from build123d import *

# Parameters (mm, degrees)
SKETCH1_W           = 250
SKETCH1_H           = 127
BOSS_EXTRUDE1_DEPTH = 6.35
SKETCH2_R           = 6.35
SKETCH2_R_2         = 3.175
SKETCH2_R_3         = 9.525
SKETCH2_R_4         = 4
SKETCH2_R_5         = 12.5
CUT_EXTRUDE1_DEPTH  = 281.480520714
CUT_EXTRUDE2_DEPTH  = 281.480520714
SKETCH9_W           = 40.64
SKETCH9_H           = 25.4
CUT_EXTRUDE3_DEPTH  = 281.480520714
FILLET1_R           = 3.96875


with BuildPart() as part:
    # Sketch1 → Boss-Extrude1 (new body)
    with BuildSketch(Plane(origin=(0, 0, 0), x_dir=(1, 0, 0), z_dir=(0, 1, 0))):
        with Locations((125, 63.5)):
            Rectangle(SKETCH1_W, SKETCH1_H)
    extrude(amount=BOSS_EXTRUDE1_DEPTH)

    # Sketch2 → Cut-Extrude1 (cut, through all)
    with BuildSketch(Plane(origin=(0, 6.35, 0), x_dir=(1, 0, 0), z_dir=(0, 1, 0))):
        with Locations(Location((237.3, 12.7, 0), (0, 0, 270))):
            Circle(SKETCH2_R)
        with Locations(Location((237.3, 114.3, 0), (0, 0, 270))):
            Circle(SKETCH2_R)
        with Locations(Location((12.7, 12.7, 0), (0, 0, 270))):
            Circle(SKETCH2_R)
        with Locations(Location((12.7, 114.3, 0), (0, 0, 270))):
            Circle(SKETCH2_R)
        with Locations(Location((43.193581925, 36.693581925, 0), (0, 0, 270))):
            Circle(SKETCH2_R_2)
        with Locations(Location((96.806418075, 36.693581925, 0), (0, 0, 270))):
            Circle(SKETCH2_R_2)
        with Locations(Location((96.806418075, 90.306418075, 0), (0, 0, 270))):
            Circle(SKETCH2_R_2)
        with Locations(Location((43.193581925, 90.306418075, 0), (0, 0, 270))):
            Circle(SKETCH2_R_2)
        with Locations(Location((70, 63.5, 0), (0, 0, 270))):
            Circle(SKETCH2_R_3)
        with Locations(Location((105.55, 19.05, 0), (0, 0, 270))):
            Circle(SKETCH2_R_4)
        with Locations(Location((194.45, 19.05, 0), (0, 0, 270))):
            Circle(SKETCH2_R_4)
        with Locations(Location((194.45, 107.95, 0), (0, 0, 270))):
            Circle(SKETCH2_R_4)
        with Locations(Location((105.55, 107.95, 0), (0, 0, 270))):
            Circle(SKETCH2_R_4)
        with Locations(Location((150, 63.5, 0), (0, 0, 270))):
            Circle(SKETCH2_R_5)
    extrude(amount=-CUT_EXTRUDE1_DEPTH, mode=Mode.SUBTRACT)

    # Sketch8 → Cut-Extrude2 (cut, through all)
    with BuildSketch(Plane(origin=(0, 6.35, 0), x_dir=(1, 0, 0), z_dir=(0, 1, 0))):
        with BuildLine():
            Line((103.01, 111.95), (118.25, 111.95))
            ThreePointArc((118.25, 111.95), (122.25, 107.95), (118.25, 103.95))
            Line((118.25, 103.95), (103.01, 103.95))
            ThreePointArc((103.01, 103.95), (99.01, 107.95), (103.01, 111.95))
        make_face()
        with BuildLine():
            Line((191.91, 111.95), (207.15, 111.95))
            ThreePointArc((207.15, 111.95), (211.15, 107.95), (207.15, 103.95))
            Line((207.15, 103.95), (191.91, 103.95))
            ThreePointArc((191.91, 103.95), (187.91, 107.95), (191.91, 111.95))
        make_face()
        with BuildLine():
            Line((103.01, 23.05), (118.25, 23.05))
            ThreePointArc((118.25, 23.05), (122.25, 19.05), (118.25, 15.05))
            Line((118.25, 15.05), (103.01, 15.05))
            ThreePointArc((103.01, 15.05), (99.01, 19.05), (103.01, 23.05))
        make_face()
        with BuildLine():
            Line((191.91, 23.05), (207.15, 23.05))
            ThreePointArc((207.15, 23.05), (211.15, 19.05), (207.15, 15.05))
            Line((207.15, 15.05), (191.91, 15.05))
            ThreePointArc((191.91, 15.05), (187.91, 19.05), (191.91, 23.05))
        make_face()
    extrude(amount=-CUT_EXTRUDE2_DEPTH, mode=Mode.SUBTRACT)

    # Sketch9 → Cut-Extrude3 (cut, through all)
    with BuildSketch(Plane(origin=(0, 6.35, 0), x_dir=(1, 0, 0), z_dir=(0, 1, 0))):
        with Locations((155.08, 63.5)):
            Rectangle(SKETCH9_W, SKETCH9_H)
    extrude(amount=-CUT_EXTRUDE3_DEPTH, mode=Mode.SUBTRACT)

    # Fillet1
    fillet1_edges = [part.edges().sort_by_distance(p)[0] for p in [
        (134.76, 3.175, -50.8),
        (134.76, 3.175, -76.2),
        (175.4, 3.175, -76.2),
        (175.4, 3.175, -50.8),
    ]]
    fillet(fillet1_edges, radius=FILLET1_R)


solid = part.part
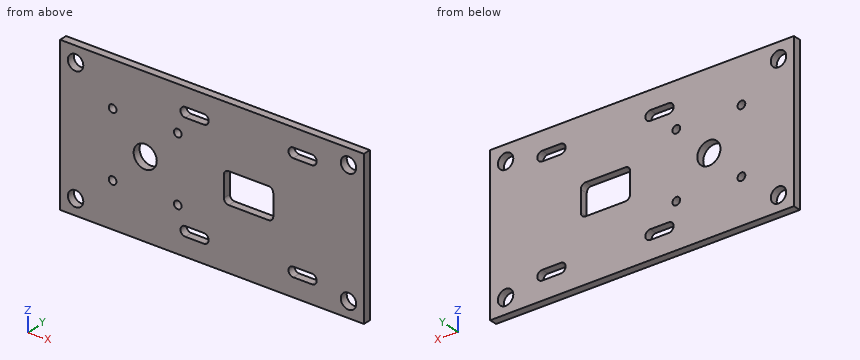
Work out the finished part from the listing and answer in its coordinate system (mm). Round coordinates to 2 decimals unless told otherwise and drop trailing zeros. Order: outer loops, then holes, each group sorted by start corner. A loop starts at its lowest first (then second) coordinate and runs counter-clockwise, first axis right, second up. Notation, with made-up numbers: M 88,-4 L 116,-4 A5 cw 116,5 Z; hole C -15,14 d1. An arc over 180 degrees is marked long. Put each result on its own line as item: value. Start each with the question number.
Q1. A flat-ended cylindrical pin translates along its axis: pin 1 (11.5 mm diameter, centred on x = 237.3, z = -114.3, fed in from -Y). Find the tip coordinate at first contact, or state that the pin passes through.
Q2. Section A-A, the plane x = 237.3 is taken. Write down the section's boundary in (y, z), and give its area (3 significant figures).
Q3. Section C-C, the plane y = 1.5 is taken. Give the number of separate pieces and of enclosed holes in the cut face, and give its area (3 significant figures).
Q4. Section B-B, the plane z = -114.3 is taken. Write down the section's boundary in (x, y), and give its area (3 significant figures).
Q5. Straight lines are drawn through the part: L1, parallel to X at y = 3.75, z = -12.7; L2, parallel to Z at x = 109.5, y = 0.75; L3, parallel to Z at x = 232, y = 2.75. For each, find the intervals that lie inside material, in ascending order. Write a range as [from, to].
Findings below:
1. pin 1: passes through
2. outline: M 0,-127 L 6.35,-127 L 6.35,-120.65 L 0,-120.65 Z; M 0,-107.95 L 6.35,-107.95 L 6.35,-19.05 L 0,-19.05 Z; M 0,-6.35 L 6.35,-6.35 L 6.35,0 L 0,0 Z
2. area: 645 mm^2
3. separate pieces: 1
3. enclosed holes: 14
3. area: 29,100 mm^2
4. outline: M 0,0 L 6.35,0 L 6.35,6.35 L 0,6.35 Z; M 19.05,0 L 230.95,0 L 230.95,6.35 L 19.05,6.35 Z; M 243.65,0 L 250,0 L 250,6.35 L 243.65,6.35 Z
4. area: 1,430 mm^2
5. L1: x = [0, 6.35], [19.05, 230.95], [243.65, 250]
5. L2: z = [-127, -111.95], [-103.95, -23.05], [-15.05, 0]
5. L3: z = [-127, -117.8], [-110.8, -16.2], [-9.2, 0]
